Geometry check sheet. Reference: the model listing, model coordinates, mm. Face numbers are marked on the shaded views. Give positions to 0.01 mm unless a question says otherwise; leave off trailing zeros. Write each loop counter-clockwise with the first axis right and the second up, starting at its lowest first coordinate (ties: lowest second). Pieces come first, ordered by that corner, then holes. Notation, with made-up numbers: (-16.5, 40) - (-7.5, 40) arc R26 ccw to (-7.5, 77) - close; hole circle Ø5 at (7, 38). An arc over 180 degrees is marked (long way). Write item = value, one per line. Start each with the question number.
(1) Thickness scan on L1, parallel to Z at x = -18, y = 1.7; L2, parallel to Z at x = -4, y = 1.35; L3, parallel to X at y = 5.1, z = -94.5. Record the ranges inside material, lowest first.
(2) Section check B-B, the plane y = 3.7. Enter the section's corners in (x, z).
(3) Section check A-A, the plane x = -18. Enter the section's corners in (y, z).
(4) Section check C-C, the plane z = -6.9. Enter the section's corners in (x, y).
(5) Draft check along Y on the marked faces 1 and 2. Enter one of: pulls with the +Y half, pulls with the -Y half, needs draft (parallel to the pull), parting line crosses it, or undercut.
(6) Section check D-D, the plane x = -4. Enter the section's corners in (y, z), plus the area to 3 significant figures.
(7) Depth check by flat-ended pin: pin 1 Ø1.7 at (x, z) = (-3, -7.5) entering from +Y; pin 2 Ø2 at (y, z) = (5, -53) entering from -X. Enter the tip coordinate at first touch or a pass-through.
Autodesk Inventor part; units mm, degrees
ref_plane "YZ Plane" through (0, 0, 0) normal (1, 0, 0) x (0, 1, 0)
ref_plane "XZ Plane" through (0, 0, 0) normal (0, 1, 0) x (-1, 0, 0)
ref_plane "XY Plane" through (0, 0, 0) normal (0, 0, 1) x (1, 0, 0)
sketch "Esquisse1" plane through (0, 0, 0) normal (0, 1, 0) x (-1, 0, 0)
  line L0 (0, 0) -> (8, 0)
  line L1 (8, -100) -> (0, -100)
  line L2 (0, -100) -> (0, 0)
  line L3 (8, 0) -> (8, -92)
  line L4 (8, -92) -> (22, -92)
  line L5 (22, -92) -> (22, -100)
  line L6 (22, -100) -> (8, -100)
  circle A0 centre (18, -96) radius 2
  circle A1 centre (7.9, -96) radius 2
  circle A2 centre (4, -6.9) radius 2.9
  circle A3 centre (4, -6.9) radius 1.25
  dimension "d0" = 8
  dimension "d1" = 100
  dimension "d2" = 8
  dimension "d5" = 10.1
  dimension "d6" = 4
  dimension "d7" = 4
  dimension "d8" = 4
  dimension "d9" = 4
  dimension "d10" = 22
  dimension "d11" = 5.8
  dimension "d12" = 4
  dimension "d13" = 4
  dimension "d15" = 4
  dimension "d17" = 2.5
extrude "Extrusion1" add sketch "Esquisse1" along normal blind 6 contours L0 L3 L4 L5 L6 L1 L2
fillet "Congé1" radius 2 5 edges at (-8, 3, 0) (0, 3, 0) (-8, 3, -92) (0, 3, -100) (-22, 3, -92)
extrude "Extrusion2" add sketch "Esquisse1" along normal blind 2 contours A2
equation "\"d2\" = d0"
equation "\"d7\" = d6"
equation "\"d8\" = 0.5 * d0"
equation "\"d12\" = d8"
equation "\"d13\" = 0.5 * d0"
properties part number "_Impression 3D"
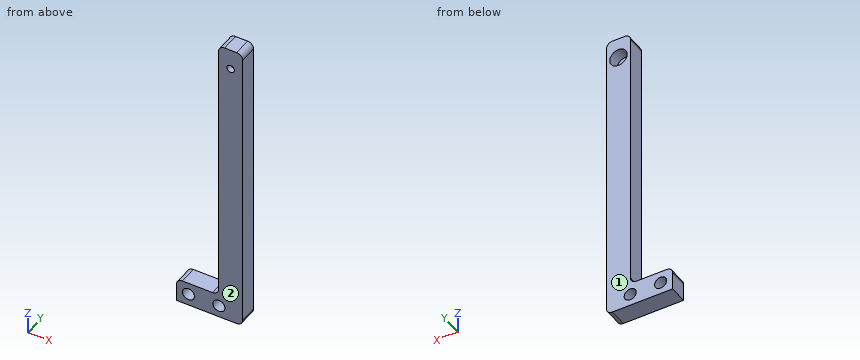
Model answer:
q1.L1 = -100 to -98, -94 to -92
q1.L2 = -100 to -8.15, -5.65 to 0
q1.L3 = -22 to -19.32, -16.68 to -9.22, -6.58 to 0
q2.outline = (-22, -100) - (-2, -100) arc R2 ccw to (0, -98) - (0, -2) arc R2 ccw to (-2, 0) - (-6, 0) arc R2 ccw to (-8, -2) - (-8, -90) arc R2 cw to (-10, -92) - (-20, -92) arc R2 ccw to (-22, -94) - close; hole circle Ø4 at (-18, -96); hole circle Ø4 at (-7.9, -96); hole circle Ø5.8 at (-4, -6.9)
q3.outline = (0, -100) - (6, -100) - (6, -98) - (0, -98) - close; (0, -94) - (6, -94) - (6, -92) - (0, -92) - close
q4.outline = (-8, 0) - (-5.25, 0) - (-5.25, 2) - (-6.9, 2) - (-6.9, 6) - (-8, 6) - close; (-2.75, 0) - (0, 0) - (0, 6) - (-1.1, 6) - (-1.1, 2) - (-2.75, 2) - close
q5.face_1 = pulls with the +Y half
q5.face_2 = pulls with the -Y half
q6.outline = (0, -100) - (6, -100) - (6, -9.8) - (2, -9.8) - (2, -8.15) - (0, -8.15) - close; (0, -5.65) - (2, -5.65) - (2, -4) - (6, -4) - (6, 0) - (0, 0) - close
q6.area = 572 mm²
q7.pin_1 = 2
q7.pin_2 = -8
